from build123d import *

# Parameters (mm, degrees)
SKETCH1_W           = 20
SKETCH1_H           = 20
BOSS_EXTRUDE1_DEPTH = 5
CIRPATTERN1_COUNT   = 4
FILLET1_R           = 2


with BuildPart() as part:
    # Sketch1 → Boss-Extrude1 (new, symmetric)
    with BuildSketch(Plane(origin=(0, 0, 0), x_dir=(0, 0, -1), z_dir=(1, 0, 0))):
        Rectangle(SKETCH1_W, SKETCH1_H)
    extrude(amount=BOSS_EXTRUDE1_DEPTH, both=True)

    # Sketch5 → Cut-Revolve3 (revolve, cut)
    with BuildSketch(Plane(origin=(0, 0, 0), x_dir=(1, 0, 0), z_dir=(0, 0.7071067811865477, 0.7071067811865475)), mode=Mode.PRIVATE) as cut_revolve3_sk:
        with BuildLine():
            Line((-5, 9.244997998), (-5, 18.244997998))
            Line((-5, 18.244997998), (5, 18.244997998))
            Line((5, 18.244997998), (5, 9.244997998))
            ThreePointArc((5, 9.244997998), (0, 11), (-5, 9.244997998))
        make_face()
    revolve(cut_revolve3_sk.sketch.rotate(Axis((-5.750529674, 0, 0), (1, 0, 0)), 135), axis=Axis((-5.750529674, 0, 0), (1, 0, 0)), mode=Mode.SUBTRACT)

    # Sketch8 → Tap Drill for M6 Tap1 (revolve, cut)
    with BuildSketch(Plane(origin=(0, 10, 0), x_dir=(0, 0, 1), z_dir=(1, 0, 0))):
        Polygon((0, 0), (0, 7.502151548), (2.5, 6), (2.5, 0), align=None)
    tap_drill_for_m6_tap1 = revolve(axis=Axis((0, 16.35, 0), (0, -1, 0)), mode=Mode.SUBTRACT)

    # CirPattern1: Tap Drill for M6 Tap1 ×4 about axis
    cirpattern1_axis = Axis((0, 0, 0), (1, 0, 0))
    for i in range(1, CIRPATTERN1_COUNT):
        add(tap_drill_for_m6_tap1.rotate(cirpattern1_axis, i * 360 / CIRPATTERN1_COUNT), mode=Mode.SUBTRACT)

    # Fillet1
    fillet1_edges = [part.edges().sort_by_distance(p)[0] for p in [
        (5, 0, -9.244997998),
        (-5, 0, -9.244997998),
    ]]
    fillet(fillet1_edges, radius=FILLET1_R)


solid = part.part
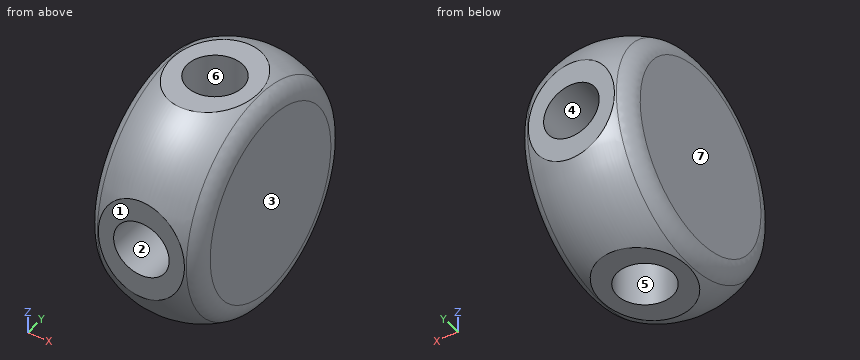
Geometry check sheet. Reference: the model listing, model coordinates, mm. Face numbers are marked on the shaded views. A direction names the side the tool comes from. Give positions to 0.01 mm unless a question says otherwise; leave off trailing zeros. Answer as a JSON object with one key per item and string values.
(1) Material ranges on line 1 (X direction, y = -6.35, z = 0); line 2 (Z direction, x = 0, y = 8.75); line 3 (Y direction, x = -0.5, z = -8.5), recorded low to high.
Report:
{"line 1": "-5 to -2.5, 2.5 to 5", "line 2": "-6.67 to -2.5, 2.5 to 6.67", "line 3": "-6.96 to -2.45, 2.45 to 6.96"}
(2) Tool access check on the marked faces 4, 5, 6 and 7. Record the directions out of +Z, -Z, +X, -X, +Y, -Y that give a thin tool (end or side, any length) a straight path to the whole face; none if there is none.
Report:
{"face 4": "+Y", "face 5": "-Z", "face 6": "+Z", "face 7": "+Z, -Z, -X, +Y, -Y"}
(3) Draft check along X on the marked faces 1, 2 and 3. Enter one of: released by +X, released by -X, zero draft, split by the parting line, or undercut.
Report:
{"face 1": "zero draft", "face 2": "undercut", "face 3": "released by +X"}
(4) Depth check by flat-ended pin: pin 1 Ø4.5 at (x, z) = (0, 0) entering from +Y; pin 2 Ø1 at (x, z) = (-2.5, -5) entering from -Y; pin 3 Ø3 at (x, y) = (0, 0) entering from +Z. Enter the tip coordinate at first touch or a pass-through.
Report:
{"pin 1": "y = 3.85", "pin 2": "y = -9.65", "pin 3": "z = 3.4"}
